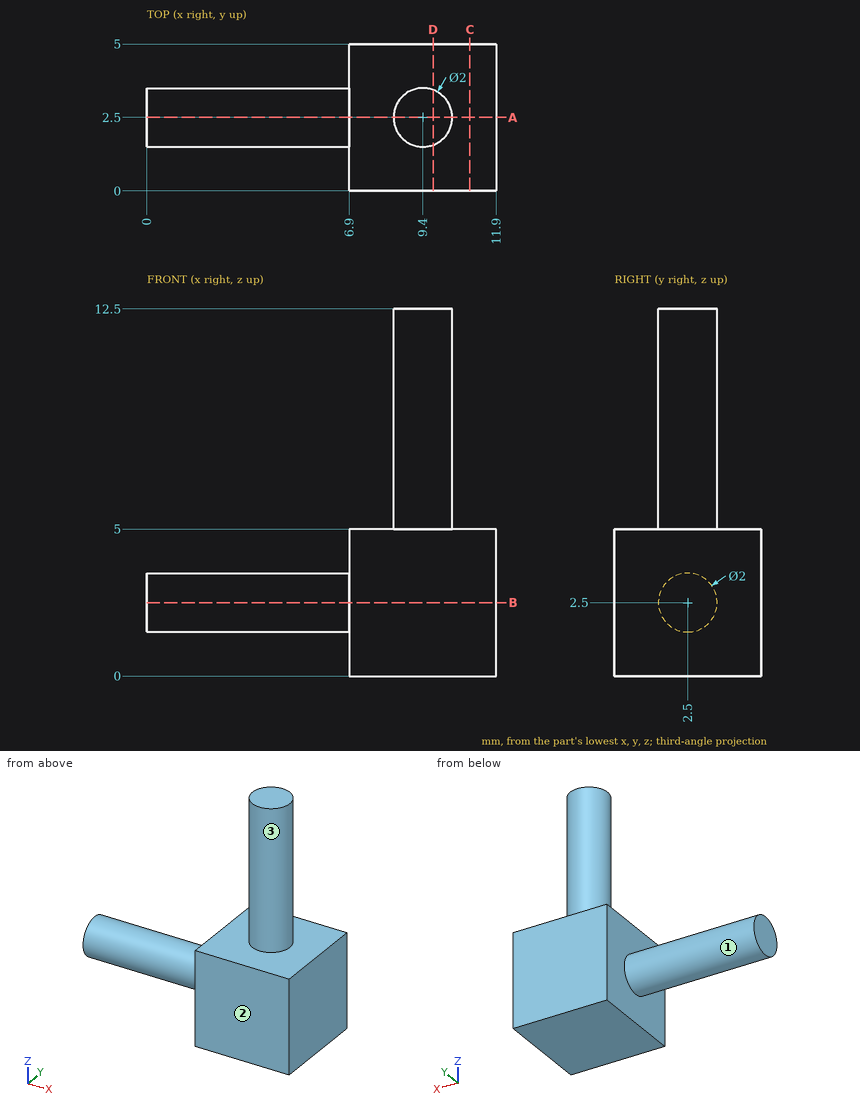
Geometry check sheet. Reference: drawing and pictorial views, mm from the part's lowest x, y, z. A direction names the side the tool comes from. Give positions to 0.01 mm unless a question says otherwise; leave off trailing zeros. Write each loop counter-clockwise with the first axis right and the second up, starting at its lowest first coordinate (ties: lowest second). Pieces come first, ordered by that corner, then holes. Notation, with made-up numbers: (-16, 10.25) - (0, 10.25) arc R12 ccw to (0, 28.25) - close; hole circle Ø1 at (9.25, 84). An arc over 180 degrees is marked (long way). Put each result on its own line as item: value.
Q1. Set-up check for the marked faces 1, 2 and 3: record each of +Z, -Z, +X, -X, +Y, -Y from which the full face is reachable in a straight line by a thin tool's end or side.
Result:
face 1: -X
face 2: +Z, -Z, +X, -X, -Y
face 3: +Z
Q2. Section check D-D on x = 9.75. Record the cut outline in (y, z), and give its area (3 significant figures).
Result:
outline: (0, 0) - (5, 0) - (5, 5) - (3.44, 5) - (3.44, 12.5) - (1.56, 12.5) - (1.56, 5) - (0, 5) - close
area: 39.1 mm2
Q3. Section check A-A on y = 2.5. Record the cut outline in (x, z), and give its area (3 significant figures).
Result:
outline: (0, 1.5) - (6.9, 1.5) - (6.9, 0) - (11.9, 0) - (11.9, 5) - (10.4, 5) - (10.4, 12.5) - (8.4, 12.5) - (8.4, 5) - (6.9, 5) - (6.9, 3.5) - (0, 3.5) - close
area: 53.8 mm2
Q4. Depth check by flat-ended pin: P1, Ø6, axis at x = 2.5, z = 5, coming from the +Y side; P2, Ø1, axis at y = 2, z = 7, coming from the +X side; P3, Ø2, axis at x = 6, y = 2.5, coming from the +Z side. Enter the tip coordinate at first touch or a pass-through.
Result:
P1: y = 3.5
P2: x = 10.4
P3: z = 5
Q5. Section check B-B on z = 2.5. Record the cut outline in (x, y).
Result:
outline: (0, 1.5) - (6.9, 1.5) - (6.9, 0) - (11.9, 0) - (11.9, 5) - (6.9, 5) - (6.9, 3.5) - (0, 3.5) - close
Q6. Scan lines: probe 1 along X at (y, z) = (4, 4); probe 2 along Z at (x, y) = (11.75, 2.2); probe 3 along Z at (x, y) = (6.25, 1.8). Record each from-to range of solid material in increasing order. Write a range as from..to.
Result:
probe 1: 6.9..11.9
probe 2: 0..5
probe 3: 1.79..3.21
Q7. Section check C-C on x = 11. Record the cut outline in (y, z), and give its area (3 significant figures).
Result:
outline: (0, 0) - (5, 0) - (5, 5) - (0, 5) - close
area: 25.0 mm2
